Check sheet for the modelled part. Datum: model origin and axes. Units: mm. Face numbers are marked on the shaded views. A direction names the side the tool comes from. Give positions to 0.01 mm unless a question says otherwise; leave off trailing zeros. Loops run counter-clockwise (first coordinate to the right, second up) from the corner with the lowest first, then second, coordinate; pieces in that order, holes last. Notation, with made-up numbers: (44.25, -23) - (72.25, -23) arc R11 ccw to (72.25, -14) - close; hole circle Ø9 at (-12.75, 15.5). An arc over 180 degrees is marked (long way). Use CSV: the item, a comma, the result in double quotes.
from build123d import *

# Parameters (mm, degrees)
BOSS_EXTRUDE1_DEPTH = 3.175
SKETCH2_R           = 2.175
CUT_EXTRUDE2_DEPTH  = 6.35
BOSS_EXTRUDE2_DEPTH = 3.175
CUT_EXTRUDE3_DEPTH  = 10
FILLET1_R           = 10
CUT_EXTRUDE4_DEPTH  = 10
SKETCH6_W           = 56.98519
SKETCH6_H           = 25.4
CUT_EXTRUDE5_DEPTH  = 71.135360158


with BuildPart() as part:
    # Sketch1 → Boss-Extrude1 (new body)
    with BuildSketch(Plane(origin=(0, 0, 0), x_dir=(1, 0, 0), z_dir=(0, 1, 0))):
        with BuildLine():
            Line((-62.844661922, 8.700177936), (13.355338078, 8.700177936))
            ThreePointArc((13.355338078, 8.700177936), (19.705338078, 2.350177936), (13.355338078, -3.999822064))
            Line((13.355338078, -3.999822064), (-62.844661922, -3.999822064))
            ThreePointArc((-62.844661922, -3.999822064), (-69.194661922, 2.350177936), (-62.844661922, 8.700177936))
        make_face()
    extrude(amount=BOSS_EXTRUDE1_DEPTH)

    # Sketch2 → Cut-Extrude2 (cut)
    with BuildSketch(Plane(origin=(0, 3.175, 0), x_dir=(1, 0, 0), z_dir=(0, 1, 0))):
        with Locations(Location((-62.844661922, 2.350177936, 0), (0, 0, 270))):
            Circle(SKETCH2_R)
        with Locations(Location((-31.094661922, 2.350177936, 0), (0, 0, 270))):
            Circle(SKETCH2_R)
        with Locations(Location((1.555338078, 2.350177936, 0), (0, 0, 270))):
            Circle(SKETCH2_R)
    extrude(amount=-CUT_EXTRUDE2_DEPTH, mode=Mode.SUBTRACT)

    # Sketch3 → Boss-Extrude2 (add)
    with BuildSketch(Plane(origin=(0, 3.175, 0), x_dir=(1, 0, 0), z_dir=(0, 1, 0))):
        with BuildLine():
            Line((13.355338078, 8.700177936), (13.355338078, 2.350177936))
            Line((13.355338078, 2.350177936), (19.705338078, 2.350177936))
            Line((19.705338078, 2.350177936), (19.705338078, 9.999403669))
            ThreePointArc((19.705338078, 9.999403669), (19.189460997, 10.874403669), (18.174088078, 10.846618776))
            ThreePointArc((18.174088078, 10.846618776), (15.930319915, 9.401611756), (13.355338078, 8.700177936))
        make_face()
    extrude(amount=-BOSS_EXTRUDE2_DEPTH)

    # Sketch4 → Cut-Extrude3 (cut)
    with BuildSketch(Plane(origin=(0, 3.175, 0), x_dir=(1, 0, 0), z_dir=(0, 1, 0))):
        with BuildLine():
            Line((19.705338078, 9.999403669), (19.705338078, -6.000596331))
            Line((19.705338078, -6.000596331), (9.205338078, -6.000596331))
            ThreePointArc((9.205338078, -6.000596331), (16.836220051, 0.436949875), (19.705338078, 9.999403669))
        make_face()
    extrude(amount=-CUT_EXTRUDE3_DEPTH, mode=Mode.SUBTRACT)

    # Fillet1
    fillet1_edges = [part.edges().sort_by_distance(p)[0] for p in [
        (12.654174153, 1.5875, 3.999822064),
    ]]
    fillet(fillet1_edges, radius=FILLET1_R)

    # Sketch5 → Cut-Extrude4 (cut)
    with BuildSketch(Plane(origin=(0, 3.175, 0), x_dir=(1, 0, 0), z_dir=(0, 1, 0))):
        Polygon((-4.314661922, 8.700177936), (-0.914661922, 8.700177936), (-1.614661922, 7.306047383), (-3.614661922, 7.306047383), align=None)
        Polygon((-9.814661922, 8.700177936), (-9.114661922, 7.306047383), (-7.114661922, 7.306047383), (-6.414661922, 8.700177936), align=None)
        Polygon((1.185338078, 8.700177936), (4.585338078, 8.700177936), (3.885338078, 7.306047383), (1.885338078, 7.306047383), align=None)
        Polygon((6.685338078, 8.700177936), (10.085338078, 8.700177936), (9.385338078, 7.306047383), (7.385338078, 7.306047383), align=None)
        Polygon((-15.314661922, 8.700177936), (-11.914661922, 8.700177936), (-12.614661922, 7.306047383), (-14.614661922, 7.306047383), align=None)
        Polygon((-20.814661922, 8.700177936), (-17.414661922, 8.700177936), (-18.114661922, 7.306047383), (-20.114661922, 7.306047383), align=None)
        Polygon((-26.314661922, 8.700177936), (-22.914661922, 8.700177936), (-23.614661922, 7.306047383), (-25.614661922, 7.306047383), align=None)
    extrude(amount=-CUT_EXTRUDE4_DEPTH, mode=Mode.SUBTRACT)

    # Sketch6 → Cut-Extrude5 (cut, through all)
    with BuildSketch(Plane(origin=(0, 3.175, 0), x_dir=(1, 0, 0), z_dir=(0, 1, 0))):
        with Locations((-40.702066922, 2.350177936)):
            Rectangle(SKETCH6_W, SKETCH6_H)
    extrude(amount=-CUT_EXTRUDE5_DEPTH, mode=Mode.SUBTRACT)


solid = part.part
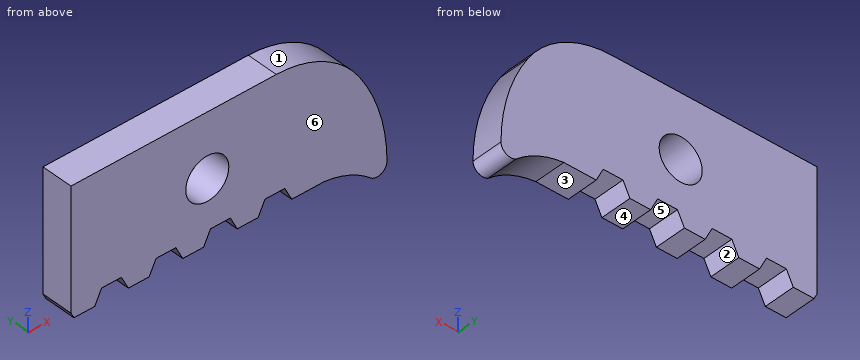
1. Sectioned sample at C-C, the plane y = 1. Record the boundary of the cut face in (x, z) (3 decimals), and give its area (3 significant figures).
Completed:
outline,"(-12.209, -8.113) - (-11.915, -8.7) - (-9.815, -8.7) - (-9.115, -7.306) - (-7.115, -7.306) - (-6.415, -8.7) - (-4.315, -8.7) - (-3.615, -7.306) - (-1.615, -7.306) - (-0.915, -8.7) - (1.185, -8.7) - (1.885, -7.306) - (3.885, -7.306) - (4.585, -8.7) - (6.685, -8.7) - (7.385, -7.306) - (9.385, -7.306) - (10.085, -8.7) - (13.355, -8.7) arc R8.75 cw to (18.174, -10.847) arc R1 ccw to (19.705, -9.999) arc R17.5 ccw to (16.952, -0.616) arc R10 ccw to (8.525, 4) - (-12.209, 4) - close; hole circle Ø4.35 at (1.555, -2.35)"
area,"350 mm²"
2. Go/stop test with flat-tipped pins: pin 1 Ø1.1 at (x, y) = (-5.5, 2.5) entering from -Z; pin 2 Ø1.6 at (x, y) = (-3, 2.5) entering from -Z; pin 3 Ø1 at (x, y) = (-8, 1.5) entering from -Z. Record where each tip stops, or that it passes through.
Completed:
pin 1,"stops at z = -8.7"
pin 2,"stops at z = -7.68"
pin 3,"stops at z = -7.31"
3. Sectioned sample at A-A, the plane z = -2.5. Record the boundary of the cut face in (x, y) (1 decimal).
Completed:
outline,"(-12.2, 0) - (-0.6, 0) - (-0.6, 3.2) - (-12.2, 3.2) - close; (3.7, 0) - (18, 0) - (18, 3.2) - (3.7, 3.2) - close"
4. Release check for a two-part mould opening along X. For the marked faces 1, 2 and 3 record: released by +X, released by -X, zero draft, split by the parting line, or undercut.
Completed:
face 1,"released by +X"
face 2,"undercut"
face 3,"zero draft"
5. Scan lines: line 1 along X through (y, z) = (2.8, -8.5); line 2 along Z through (x, y) = (-2, 2.7); line 3 along Z through (x, y) = (6.5, 2.6). Record each from-to range of solid material in increasing order.
Completed:
line 1,"x = -12.02 to -9.71, -6.52 to -4.21, -1.02 to 1.29, 4.48 to 6.79, 9.98 to 19.64"
line 2,"z = -7.31 to 4"
line 3,"z = -8.7 to 4"
6. Set-up check for the marked faces 4, 5 and 6: record each of +Z, -Z, +X, -X, +Y, -Y from which the full face is reachable in a straight line by a thin tool's end or side.
Completed:
face 4,"-Z, -X, +Y, -Y"
face 5,"-Z, +Y, -Y"
face 6,"+Z, -Z, +X, -X, -Y"
7. Sectioned sample at D-D, the plane x = 8. Record the boundary of the cut face in (y, z) (3 decimals), and give its area (3 significant figures).
Completed:
outline,"(0, -7.306) - (3.175, -7.306) - (3.175, 4) - (0, 4) - close"
area,"35.9 mm²"
8. Sectioned sample at B-B, the plane x = 3. Record the boundary of the cut face in (y, z) (3 decimals).
Completed:
outline,"(0, -7.306) - (3.175, -7.306) - (3.175, -3.976) - (0, -3.976) - close; (0, -0.724) - (3.175, -0.724) - (3.175, 4) - (0, 4) - close"
